CAD build for the part. Positions are in the model's coordinates, mm. Coordinates: 2 decimals unless noted, no trailing zeros.
```python
from build123d import *

# Parameters (mm, degrees)
SKETCH_1_W            = 500
SKETCH_1_H            = 220
EXTRUDE_1_DEPTH       = 50
CUT_EXTRUDE_1_DEPTH   = 65
SKETCH_3_W            = 24.993501938
SKETCH_3_H            = 24.754329671
EXTRUDE_2_DEPTH       = 50
SKETCH_4_W            = 557.488309353
SKETCH_4_H            = 263.064748201
SKETCH_4_W_2          = 497.488309353
SKETCH_4_H_2          = 203.064748201
CUT_EXTRUDE_1_2_DEPTH = 84
SCALE_1_SCALE         = 1.5
SKETCH_8_W            = 822.232464029
SKETCH_8_H            = 353.597122302
SKETCH_8_W_2          = 722.232464029
SKETCH_8_H_2          = 253.597122302
CUT_EXTRUDE_2_DEPTH   = 180


with BuildPart() as part:
    # Эскиз1 → Бобышка-Вытянуть1 (new body)
    with BuildSketch(Plane.XY):
        with Locations((315.178539616, -203.237931197)):
            Rectangle(SKETCH_1_W, SKETCH_1_H)
        Polygon((203.546220768, -131.339893042), (185.513397027, -144.433418222), (140.884350264, -144.433418222), (131.736418609, -131.339893042), align=None, mode=Mode.SUBTRACT)
        Polygon((159.677066091, -260.404641243), (87.867263933, -260.404641243), (105.900087674, -247.311116064), (150.529134437, -247.311116064), align=None, mode=Mode.SUBTRACT)
        Polygon((116.392443789, -207.416781531), (103.766544509, -244.593040524), (85.938307098, -258.534137646), (104.994062494, -202.419029733), (111.160879041, -198.678022538), align=None, mode=Mode.SUBTRACT)
        Polygon((109.933361055, -187.922626855), (128.287677602, -133.911835488), (136.67571717, -147.706799517), (124.225177602, -184.41543261), (113.060609257, -193.066511747), align=None, mode=Mode.SUBTRACT)
        Polygon((181.158630839, -203.997267143), (162.86276753, -257.832698797), (154.445501343, -244.066961387), (166.92526753, -207.299875056), (178.20674235, -198.678022538), align=None, mode=Mode.SUBTRACT)
        Polygon((174.874907818, -183.947806711), (187.354674005, -147.239173618), (205.124458178, -133.444209589), (186.770141631, -187.455000956), (180.106472566, -193.066511747), align=None, mode=Mode.SUBTRACT)
        Polygon((172.098379041, -189.325504553), (176.833091271, -195.872267143), (167.626706379, -202.419029733), (119.695051703, -202.419029733), (114.931112854, -195.872267143), (124.166724365, -189.325504553), align=None, mode=Mode.SUBTRACT)
        Polygon((188.173019329, -260.404641243), (192.615465372, -247.311116064), (205.708990552, -247.311116064), (201.266544509, -260.404641243), align=None, mode=Mode.SUBTRACT)
        Polygon((220.585339473, -165.00895779), (225.057012134, -151.91543261), (238.150537314, -151.91543261), (233.678864652, -165.00895779), align=None, mode=Mode.SUBTRACT)
        Polygon((347.574997746, -131.339893042), (329.542174005, -144.433418222), (284.913127242, -144.433418222), (275.765195588, -131.339893042), align=None, mode=Mode.SUBTRACT)
        Polygon((303.70584307, -260.404641243), (231.896040911, -260.404641243), (249.928864652, -247.311116064), (294.557911415, -247.311116064), align=None, mode=Mode.SUBTRACT)
        Polygon((260.421220768, -207.416781531), (247.795321487, -244.593040524), (229.967084077, -258.534137646), (249.022839473, -202.419029733), (255.189656019, -198.678022538), align=None, mode=Mode.SUBTRACT)
        Polygon((253.962138034, -187.922626855), (272.31645458, -133.911835488), (280.704494149, -147.706799517), (268.25395458, -184.41543261), (257.089386235, -193.066511747), align=None, mode=Mode.SUBTRACT)
        Polygon((325.187407818, -203.997267143), (306.891544509, -257.832698797), (298.474278321, -244.066961387), (310.954044509, -207.299875056), (322.235519329, -198.678022538), align=None, mode=Mode.SUBTRACT)
        Polygon((318.903684796, -183.947806711), (331.383450983, -147.239173618), (349.153235156, -133.444209589), (330.798918609, -187.455000956), (324.135249545, -193.066511747), align=None, mode=Mode.SUBTRACT)
        Polygon((316.127156019, -189.325504553), (320.86186825, -195.872267143), (311.655483357, -202.419029733), (263.723828681, -202.419029733), (258.959889832, -195.872267143), (268.195501343, -189.325504553), align=None, mode=Mode.SUBTRACT)
        Polygon((446.711688393, -131.339893042), (428.678864652, -144.433418222), (384.04981789, -144.433418222), (374.901886235, -131.339893042), align=None, mode=Mode.SUBTRACT)
        Polygon((402.842533717, -260.404641243), (331.032731559, -260.404641243), (349.0655553, -247.311116064), (393.694602063, -247.311116064), align=None, mode=Mode.SUBTRACT)
        Polygon((359.557911415, -207.416781531), (346.932012134, -244.593040524), (329.103774724, -258.534137646), (348.15953012, -202.419029733), (354.326346667, -198.678022538), align=None, mode=Mode.SUBTRACT)
        Polygon((353.098828681, -187.922626855), (371.453145228, -133.911835488), (379.841184796, -147.706799517), (367.390645228, -184.41543261), (356.226076883, -193.066511747), align=None, mode=Mode.SUBTRACT)
        Polygon((424.324098465, -203.997267143), (406.028235156, -257.832698797), (397.610968969, -244.066961387), (410.090735156, -207.299875056), (421.372209976, -198.678022538), align=None, mode=Mode.SUBTRACT)
        Polygon((418.040375444, -183.947806711), (430.520141631, -147.239173618), (448.289925804, -133.444209589), (429.935609257, -187.455000956), (423.271940192, -193.066511747), align=None, mode=Mode.SUBTRACT)
        Polygon((415.263846667, -189.325504553), (419.998558897, -195.872267143), (410.792174005, -202.419029733), (362.860519329, -202.419029733), (358.09658048, -195.872267143), (367.332191991, -189.325504553), align=None, mode=Mode.SUBTRACT)
        Polygon((545.848379041, -131.339893042), (527.8155553, -144.433418222), (483.186508537, -144.433418222), (474.038576883, -131.339893042), align=None, mode=Mode.SUBTRACT)
        Polygon((501.979224365, -260.404641243), (430.169422206, -260.404641243), (448.202245947, -247.311116064), (492.83129271, -247.311116064), align=None, mode=Mode.SUBTRACT)
        Polygon((458.694602063, -207.416781531), (446.068702782, -244.593040524), (428.240465372, -258.534137646), (447.296220768, -202.419029733), (453.463037314, -198.678022538), align=None, mode=Mode.SUBTRACT)
        Polygon((452.235519329, -187.922626855), (470.589835875, -133.911835488), (478.977875444, -147.706799517), (466.527335875, -184.41543261), (455.36276753, -193.066511747), align=None, mode=Mode.SUBTRACT)
        Polygon((523.460789113, -203.997267143), (505.164925804, -257.832698797), (496.747659616, -244.066961387), (509.227425804, -207.299875056), (520.508900624, -198.678022538), align=None, mode=Mode.SUBTRACT)
        Polygon((517.177066091, -183.947806711), (529.656832278, -147.239173618), (547.426616451, -133.444209589), (529.072299904, -187.455000956), (522.408630839, -193.066511747), align=None, mode=Mode.SUBTRACT)
        Polygon((514.400537314, -189.325504553), (519.135249545, -195.872267143), (509.928864652, -202.419029733), (461.997209976, -202.419029733), (457.233271127, -195.872267143), (466.468882638, -189.325504553), align=None, mode=Mode.SUBTRACT)
    extrude(amount=EXTRUDE_1_DEPTH)

    # Эскиз2 → Cut-Extrude 1 (cut)
    with BuildSketch(Plane.XY.offset(50)):
        Polygon((225.057012134, -151.91543261), (238.150537314, -151.91543261), (233.678864652, -165.00895779), (220.585339473, -165.00895779), align=None)
        Polygon((199.643902872, -226.731116064), (212.737428052, -226.731116064), (208.26575539, -239.824641243), (195.17223021, -239.824641243), align=None)
    extrude(amount=-CUT_EXTRUDE_1_DEPTH, mode=Mode.SUBTRACT)

    # Эскиз3 → Бобышка-Вытянуть2 (add)
    with BuildSketch(Plane.XY.offset(50)):
        with Locations((196.457377331, -256.289777907)):
            Rectangle(SKETCH_3_W, SKETCH_3_H)
    extrude(amount=-EXTRUDE_2_DEPTH)

    # Эскиз4 → Cut-Extrude 1 2 (cut)
    with BuildSketch(Plane.XY.offset(50)):
        with Locations((316.682461775, -195.872267142)):
            Rectangle(SKETCH_4_W, SKETCH_4_H)
        with Locations((316.682461775, -195.872267142)):
            Rectangle(SKETCH_4_W_2, SKETCH_4_H_2, mode=Mode.SUBTRACT)
    extrude(amount=-CUT_EXTRUDE_1_2_DEPTH, mode=Mode.SUBTRACT)


with BuildPart() as part_1:
    # Масштаб1: scaled about (314.289349403, -195.861916492, 25)
    add(part.part.scale(SCALE_1_SCALE).moved(Location((-157.144674702, 97.930958246, -12.5))))

    # Эскиз8 → Вырез-Вытянуть-Тонкостенный2 (cut)
    with BuildSketch(Plane.XY.offset(62.5)):
        with Locations((317.879017961, -195.877442468)):
            Rectangle(SKETCH_8_W, SKETCH_8_H)
        with Locations((317.879017961, -195.877442468)):
            Rectangle(SKETCH_8_W_2, SKETCH_8_H_2, mode=Mode.SUBTRACT)
    extrude(amount=-CUT_EXTRUDE_2_DEPTH, mode=Mode.SUBTRACT)


solid = part_1.part
```
Item 1: Saw through at A-A, the plane y = -227. State how many separate pieces and enclosed holes the cut face has, and give its area (3 significant figures).
Item 2: Wall check: line 1 along Y through (x, z) = (422, 53); line 2 along X through (y, z) = (-100, 35); line 3 along Y through (x, z) = (184.5, 9.5). Give the ranges that are in metal, low to high.
Item 3: Two-plate mould, pull along Y, no slides. Class faces 1 (the flat face through (313, -166, 62.5)), 2 (the flat face through (588.87, -282.72, 24.48)): +Y half, -Y half, draft (parallel to the pull), parting line (faces both ways), or undercut.
Working result:
1. separate pieces: 9
1. enclosed holes: 0
1. area: 42,400 mm2
2. line 1: y = -322.68 to -292.68, -273.04 to -205.7, -186.06 to -118.72, -99.08 to -69.08
2. line 2: x = -43.24 to 41.1, 146.91 to 257.15, 362.95 to 405.85, 511.65 to 554.56, 660.36 to 679
2. line 3: y = -322.68 to -149.58, -129.94 to -69.08
3. face 1: draft
3. face 2: undercut
